Could you check a few things on this drawing? It's one solid part, dimensions in mm from its lowest x, y, z. A direction names the side the tool comes from. Round coordinates to 2 decimals unless told otherwise and drop trailing zeros. Write each loop counter-clockwise with the first axis right and the second up, starting at its lowest first coordinate (ties: lowest second). Pieces come first, ordered by that corner, then holes. Notation, with made-up numbers: (36, 31) -> (61, 31) arc R9 cw to (61, 48) -> close; hole circle Ø6 at (23, 43.25). An arc over 180 degrees is marked (long way). Answer in a Markdown table with one row per item.
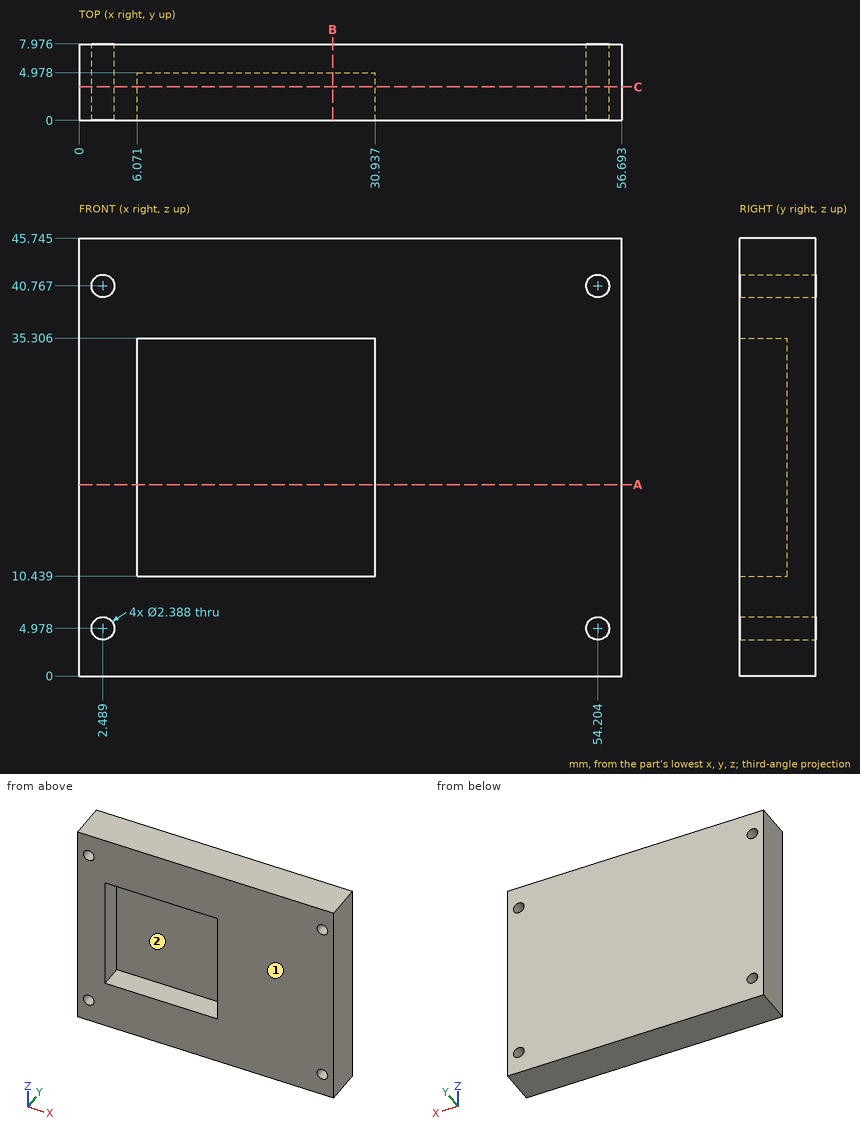
1) I want a section at B-B, the plane x = 26.5. List the corners of the cut face in (y, z) for me (1 decimal).
Response:
| item | result |
|---|---|
| outline | (0, 0) -> (8, 0) -> (8, 45.7) -> (0, 45.7) -> (0, 35.3) -> (5, 35.3) -> (5, 10.4) -> (0, 10.4) -> close |
2) I want a section at C-C, the plane y = 3.5. List the corners of the cut face in (x, z) for me (1 decimal).
Response:
| item | result |
|---|---|
| outline | (0, 0) -> (56.7, 0) -> (56.7, 45.7) -> (0, 45.7) -> close; hole circle Ø2.4 at (2.5, 5); hole circle Ø2.4 at (2.5, 40.8); hole (6.1, 10.4) -> (30.9, 10.4) -> (30.9, 35.3) -> (6.1, 35.3) -> close; hole circle Ø2.4 at (54.2, 5); hole circle Ø2.4 at (54.2, 40.8) |
3) I need wall thicknesses on line 1 (X direction, y = 4.75, z = 35); line 2 (Z direction, x = 8.5, y = 3) (1 decimal); line 3 (X direction, y = 3.75, z = 6) (1 decimal). Which ranges of each line are inside material? Lowest first, please. Write a range as [from, to].
Response:
| item | result |
|---|---|
| line 1 | x = [0, 6.07], [30.94, 56.69] |
| line 2 | z = [0, 10.4], [35.3, 45.7] |
| line 3 | x = [0, 1.9], [3.1, 53.6], [54.8, 56.7] |
4) Which directions (+Z, -Z, +X, -X, +Y, -Y) give clear straight access to the entire face, cutting with the end or side of a thin tool? Please do the marked faces 1 and 2.
Response:
| item | result |
|---|---|
| face 1 | +Z, -Z, +X, -X, -Y |
| face 2 | -Y |
5) I want a section at A-A, the plane z = 20. List the corners of the cut face in (x, y) for me (1 decimal), and give its area (3 significant figures).
Response:
| item | result |
|---|---|
| outline | (0, 0) -> (6.1, 0) -> (6.1, 5) -> (30.9, 5) -> (30.9, 0) -> (56.7, 0) -> (56.7, 8) -> (0, 8) -> close |
| area | 328 mm^2 |
